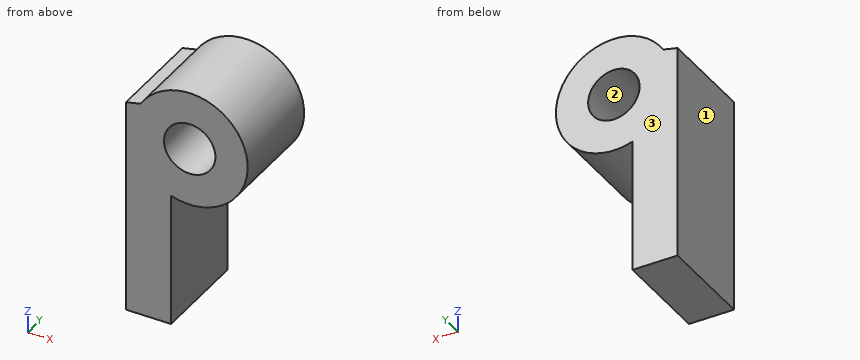
```python
from build123d import *

# Parameters (mm, degrees)
F0_R     = 6.562201
F1_DEPTH = 25


with BuildPart() as f1:
    # F0 (on Front) → F1 (new body)
    with BuildSketch(Plane.XZ):
        with BuildLine():
            Line((16.947664, 43.057742), (13.250001, 42.2474))
            Line((13.250001, 42.2474), (13.250001, -12.752604))
            Line((13.250001, -12.752604), (24.750002, -12.752604))
            Line((24.750002, -12.752604), (24.750002, 21.247396))
            ThreePointArc((24.750002, 21.247396), (43.41997, 40.227069), (16.947664, 43.057742))
        make_face()
        with Locations((29.500002, 35.2474)):
            Circle(F0_R, mode=Mode.SUBTRACT)
    extrude(amount=F1_DEPTH)


solid = f1.part
```
Input: part model. Units: mm. Frame: model coordinates. Face numbers are marked on the shaded views. Give positions to 0.01 mm unless a question says otherwise; leave off trailing zeros. Order: outer loops, then holes, each group sorted by start corner. A loop starts at its lowest first (then second) coordinate and runs counter-clockwise, first axis right, second up. Notation, with made-up numbers: (13.25, 14.5) - (68.25, 14.5) arc R22 cw to (68.25, 41.5) - close; hole circle Ø11 at (-34, 6). An arc over 180 degrees is marked (long way). One line per item, written item: value.
1. Cut plane D-D, the plane z = 18. Output: boundary loops of the cut face in (x, y).
Determined:
outline: (13.25, -25) - (24.75, -25) - (24.75, 0) - (13.25, 0) - close
2. Draft query along X for the marked faces 1, 2 and 3. Return one class per face: released by +X, released by -X, zero draft, split by the parting line, or undercut.
Determined:
face 1: released by -X
face 2: undercut
face 3: zero draft
3. Cut plane C-C, the plane x = 15.5. Output: boundary loops of the cut face in (y, z).
Determined:
outline: (-25, -12.75) - (0, -12.75) - (0, 42.74) - (-25, 42.74) - close
4. Pin query (flat end, axial travel): pin 1 Ø7.5 at (y, z) = (-10, 1.5) entering from +X; pin 2 Ø1.5 at (x, y) = (29, -16) entering from -Z; pin 3 Ø10 at (y, z) = (-8.5, 24.5) entering from +X; pin 4 Ø8 at (x, z) = (29.5, 35.25) entering from -Y. Return the tip coordinate at first contact, or that it passes through.
Determined:
pin 1: x = 24.75
pin 2: z = 20.46
pin 3: x = 43.12
pin 4: through
5. Line query: probe 1 along Z at (x, y) = (29.5, -1.5); probe 2 along X at (y, z) = (-19, -10); probe 3 along Z at (x, y) = (26.5, -14.5). Output: solid intervals per line, ascending.
Determined:
probe 1: 20.46 to 28.69, 41.81 to 50.03
probe 2: 13.25 to 24.75
probe 3: 20.77 to 29.41, 41.08 to 49.72
6. Cut plane B-B, the plane y = -12.75. Output: boundary loops of the cut face in (x, z).
Determined:
outline: (13.25, -12.75) - (24.75, -12.75) - (24.75, 21.25) arc R14.78 ccw (long way) to (16.95, 43.06) - (13.25, 42.25) - close; hole circle Ø13.12 at (29.5, 35.25)
7. Cut plane A-A, the plane z = 30. Output: boundary loops of the cut face in (x, y), and give its area (3 significant figures).
Determined:
outline: (13.25, -25) - (25.56, -25) - (25.56, 0) - (13.25, 0) - close; (33.44, -25) - (43.32, -25) - (43.32, 0) - (33.44, 0) - close
area: 555 mm2
